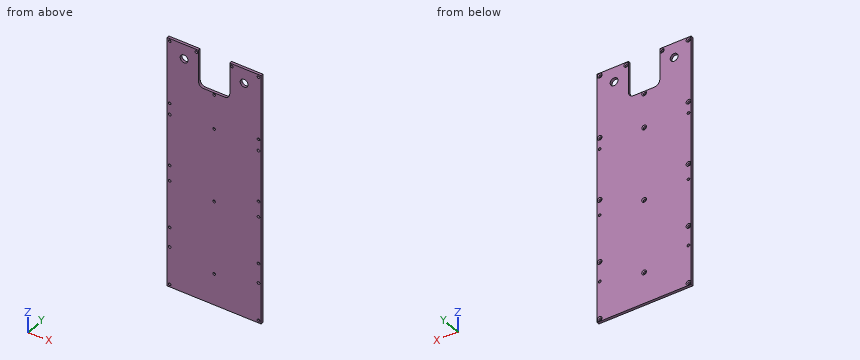
```python
from build123d import *

# Parameters (mm, degrees)
EXTRUDE1_DEPTH                                    = 3.175
CSK_FOR_4_FLAT_HEAD_MACHINE_SCREW_100_D           = 3.2639
CSK_FOR_4_FLAT_HEAD_MACHINE_SCREW_100_CSINK_D     = 5.715
CSK_FOR_4_FLAT_HEAD_MACHINE_SCREW_100_CSINK_ANGLE = 100
FILLET1_R                                         = 6.35
FILLET2_R                                         = 6.35
SKETCH4_R                                         = 4.7625
CUT_EXTRUDE1_DEPTH                                = 4.175
SKETCH5_W                                         = 114.3
SKETCH5_H                                         = 19.05
CUT_EXTRUDE2_DEPTH                                = 4.175
F_4_CLEARANCE_HOLE1_D                             = 3.2639
F_4_CLEARANCE_HOLE1_DEPTH                         = 6.35
F_4_CLEARANCE_HOLE1_TIP                           = 0.980574487


with BuildPart() as part:
    # Sketch1 → Extrude1 (new body)
    with BuildSketch(Plane(origin=(0, 0, 0), x_dir=(1, 0, 0), z_dir=(0, 1, 0))):
        Polygon((-57.15, -171.45), (-57.15, 152.4), (57.15, 152.4), (57.15, -171.45), (19.05, -171.45), (19.05, -107.95), (-19.05, -107.95), (-19.05, -171.45), align=None)
    extrude(amount=EXTRUDE1_DEPTH)

    # CSK for #4 Flat Head Machine Screw (100)1 (through all)
    with Locations(Plane(origin=(-53.975, 3.175, -149.225), x_dir=(0, 0, 1), z_dir=(0, 1, 0))):
        with Locations((0, 0), (0, 107.95), (298.45, 107.95), (298.45, 75.565), (254.635, 53.975), (298.45, 32.385), (298.45, 0), (69.85, 0), (146.05, 0), (222.25, 0), (222.25, 107.95), (146.05, 107.95), (69.85, 107.95), (34.925, 53.975), (212.725, 53.975), (123.825, 53.975)):
            CounterSinkHole(CSK_FOR_4_FLAT_HEAD_MACHINE_SCREW_100_D / 2, CSK_FOR_4_FLAT_HEAD_MACHINE_SCREW_100_CSINK_D / 2, counter_sink_angle=CSK_FOR_4_FLAT_HEAD_MACHINE_SCREW_100_CSINK_ANGLE)

    # Fillet1
    fillet1_edges = [part.edges().sort_by_distance(p)[0] for p in [
        (-19.05, 1.5875, 107.95),
    ]]
    fillet(fillet1_edges, radius=FILLET1_R)

    # Fillet2
    fillet2_edges = [part.edges().sort_by_distance(p)[0] for p in [
        (19.05, 1.5875, 107.95),
    ]]
    fillet(fillet2_edges, radius=FILLET2_R)

    # Sketch4 → Cut-Extrude1 (cut, through all)
    with BuildSketch(Plane(origin=(0, 3.175, 0), x_dir=(-1, 0, 0), z_dir=(0, 1, 0))):
        with Locations((36.5125, 134.62)):
            Circle(SKETCH4_R)
        with Locations((-36.5125, 134.62)):
            Circle(SKETCH4_R)
    extrude(amount=-CUT_EXTRUDE1_DEPTH, mode=Mode.SUBTRACT)

    # Sketch5 → Cut-Extrude2 (cut, through all)
    with BuildSketch(Plane(origin=(0, 3.175, 0), x_dir=(-1, 0, 0), z_dir=(0, 1, 0))):
        with Locations((0, 161.925)):
            Rectangle(SKETCH5_W, SKETCH5_H)
    extrude(amount=-CUT_EXTRUDE2_DEPTH, mode=Mode.SUBTRACT)

    # #4 Clearance Hole1
    with Locations(Plane(origin=(-53.975, 3.175, -103.378), x_dir=(0, 0, 1), z_dir=(0, 1, 0))):
        with Locations((0, 0), (0, 107.95), (81.28, 107.95), (81.28, 0), (162.56, 0), (162.56, 107.95)):
            Hole(F_4_CLEARANCE_HOLE1_D / 2, depth=F_4_CLEARANCE_HOLE1_DEPTH)
            with Locations((0, 0, -(F_4_CLEARANCE_HOLE1_DEPTH + F_4_CLEARANCE_HOLE1_TIP / 2))):  # 118° drill point
                Cone(0, F_4_CLEARANCE_HOLE1_D / 2, F_4_CLEARANCE_HOLE1_TIP, mode=Mode.SUBTRACT)


solid = part.part
```
Could you check a few things on this model? Use its own coordinates, in mm. Round coordinates to 2 decimals unless told otherwise and drop trailing zeros. Write each question's results on one line, items separated by ' | '. Start each with the question number.
1. I need wall thicknesses on L1, parallel to X at y = 2.75, z = 140; L2, parallel to Z at x = 22, y = 2.15; L3, parallel to X at y = 2.7, z = -5. Which ranges of each line are inside material? Lowest first, please. Write a range as from..to.
2. I'm going to push flat-ended pins straight in: pin 1 Ø5 at (x, z) = (53.975, -79.375) entering from +Y (3 decimals); pin 2 Ø4 at (x, z) = (-53.975, -3.175) entering from +Y. Where does each tip first touch, or does it pass through?
3. Imagine slicing it at A-A on y = 0.85. Count the separate pieces of the cut face and the enclosed holes in it, and give its area (3 significant figures).
Result sheet:
1) L1: x = -57.15..-19.05, 19.05..57.15 | L2: z = -152.4..147.64, 150.81..152.4 | L3: x = -57.15..-55.36, -52.59..52.59, 55.36..57.15
2) pin 1: stops at y = 2.875 | pin 2: stops at y = 2.46
3) separate pieces: 1 | enclosed holes: 24 | area: 32,800 mm^2
